Autodesk Inventor part; units mm, degrees
ref_plane "Arbeitsebene3" through (-32.75, 5, -38) normal (0, 1, 0) x (0, 0, 1)
ref_plane "YZ Plane" through (0, 0, 0) normal (1, 0, 0) x (0, 1, 0)
ref_plane "XZ Plane" through (0, 0, 0) normal (0, 1, 0) x (-1, 0, 0)
sketch "Skizze1" plane through (0, 0, 0) normal (0, 1, 0) x (-1, 0, 0)
  line L0 (-37.75, -63.9) -> (37.75, -63.9)
  line L1 (42.75, -58.9) -> (42.75, 58.9)
  line L2 (37.75, 63.9) -> (-37.75, 63.9)
  line L3 (-42.75, 58.9) -> (-42.75, -58.9)
  line L4 (-42.75, -63.9) -> (42.75, 63.9) construction
  line L5 (42.75, -63.9) -> (-42.75, 63.9) construction
  arc A0 (42.75, 58.9) -> (37.75, 63.9) centre (37.75, 58.9) ccw
  arc A1 (-37.75, 63.9) -> (-42.75, 58.9) centre (-37.75, 58.9) ccw
  arc A2 (-42.75, -58.9) -> (-37.75, -63.9) centre (-37.75, -58.9) ccw
  arc A3 (37.75, -63.9) -> (42.75, -58.9) centre (37.75, -58.9) ccw
  point P0 (0, 0)
  dimension "d0" = 85.5
  dimension "d1" = 127.8
  dimension "d2" = 5
extrude "Extrusion1" add sketch "Skizze1" along normal blind 10
ref_plane "Arbeitsebene1" through (37.75, 0, 0) normal (0, 0, -1) x (-1, 0, 0)
ref_plane "Arbeitsebene2" through (0, 0, 58.9) normal (1, 0, 0) x (0, 0, -1)
sketch "Skizze2" plane through (0, 10, 0) normal (0, 1, 0) x (1, 0, 0)
  line L0 (-12.95, 38) -> (-38.75, 38)
  line L1 (-38.75, -38) -> (-12.95, -38)
  line L2 (-12.95, -38) -> (-12.95, -2.5)
  line L3 (-38.75, 38) -> (-38.75, -38)
  line L4 (-38.75, -38) -> (-12.95, -38)
  line L5 (-12.95, -38) -> (-12.95, 38)
  line L6 (-12.95, 38) -> (-38.75, 38)
  line L7 (-38.75, 38) -> (-38.75, -38)
  line L8 (-11.95, 39) -> (-11.95, -39)
  line L9 (-11.95, -39) -> (-39.75, -39)
  line L10 (-39.75, -39) -> (-39.75, 39)
  line L11 (-39.75, 39) -> (-11.95, 39)
  line L12 (-38.75, 38) -> (-38.75, 39)
  line L13 (-38.75, -38) -> (-38.75, -39)
  point P0 (0, 0)
  dimension "d5" = 1
extrude "Extrusion2" cut sketch "Skizze2" against normal through all contours L5 L2 L1 L3 L0 | L0 L12 L11 L8 L9 L13 L1 L2 L5
ref_plane "Arbeitsebene3" through (-32.75, 5, -38) normal (0, 1, 0) x (0, 0, 1)
sketch "Skizze3" plane through (0, 10, 0) normal (0, 1, 0) x (1, 0, 0)
  line L0 (-11.95, -39) -> (-38.75, -39)
  line L1 (-38.75, 39) -> (-11.95, 39)
  line L2 (-11.95, 39) -> (-11.95, -39)
  arc A0 (-37.75, 63.9) -> (-42.75, 58.9) centre (-37.75, 58.9) ccw
  line L3 (-42.75, 58.9) -> (-42.75, -58.9)
  arc A1 (-42.75, -58.9) -> (-37.75, -63.9) centre (-37.75, -58.9) ccw
  line L4 (-37.75, -63.9) -> (37.75, -63.9)
  arc A2 (37.75, -63.9) -> (42.75, -58.9) centre (37.75, -58.9) ccw
  line L5 (42.75, -58.9) -> (42.75, 58.9)
  arc A3 (42.75, 58.9) -> (37.75, 63.9) centre (37.75, 58.9) ccw
  line L6 (37.75, 63.9) -> (-37.75, 63.9)
  line L7 (-39.75, -39) -> (-39.75, 39)
  line L8 (-11.95, 39) -> (-11.95, -39)
  line L9 (-39.75, -39) -> (-11.95, -39)
  line L10 (-11.95, -39) -> (-11.95, -34)
  line L11 (-11.95, -34) -> (-39.75, -34)
  line L12 (-39.75, -34) -> (-39.75, -39)
  line L13 (-39.75, 39) -> (-11.95, 39)
  line L14 (-11.95, 39) -> (-11.95, 34)
  line L15 (-11.95, 34) -> (-39.75, 34)
  line L16 (-39.75, 34) -> (-39.75, 39)
  line L17 (-38.75, -39) -> (-38.75, 39)
  point P0 (0, 0)
  point P1 (-11.95, -34)
  point P2 (-38.75, 34)
  point P3 (-38.75, -34)
  dimension "d8" = 27.8
  dimension "d9" = 5
  dimension "d10" = 5
extrude "Extrusion3" add sketch "Skizze3" against normal blind 1 contours L0 L17 L11 L2 | L15 L17 L1 L2
sketch "Skizze4" plane through (0, 0, 0) normal (0, -1, 0) x (1, 0, 0)
  line L0 (-38.75, 39) -> (-11.95, 39)
  line L1 (-11.95, 39) -> (-11.95, -39)
  line L2 (-11.95, -39) -> (-38.75, -39)
  arc A0 (-42.75, -58.9) -> (-37.75, -63.9) centre (-37.75, -58.9) ccw
  line L3 (37.75, -63.9) -> (-37.75, -63.9)
  arc A1 (37.75, -63.9) -> (42.75, -58.9) centre (37.75, -58.9) ccw
  line L4 (42.75, 58.9) -> (42.75, -58.9)
  arc A2 (42.75, 58.9) -> (37.75, 63.9) centre (37.75, 58.9) ccw
  line L5 (-37.75, 63.9) -> (37.75, 63.9)
  arc A3 (-37.75, 63.9) -> (-42.75, 58.9) centre (-37.75, 58.9) ccw
  line L6 (-42.75, -58.9) -> (-42.75, 58.9)
  line L7 (-11.95, -34) -> (-11.95, 34)
  line L8 (-11.95, 34) -> (12.75, 34)
  line L9 (12.75, 34) -> (12.75, -34)
  line L10 (12.75, -34) -> (-11.95, -34)
  line L11 (-11.95, -34) -> (-11.95, 34)
  line L12 (-2.45, 7.5) -> (-2.45, -8)
  line L13 (12.75, -34.1) -> (12.75, -39.1)
  line L14 (-38.75, -39) -> (-38.75, 39)
  point P0 (0, 0)
  point P1 (-11.95, -34)
  dimension "d14" = 5
  dimension "d15" = 5
  dimension "d44" = 0
extrude "Extrusion4" cut sketch "Skizze4" against normal through all contours L8 L9 L10 L1
sketch "Skizze5" plane through (0, 0, 0) normal (0, -1, 0) x (1, 0, 0)
  arc A0 (-42.75, -58.9) -> (-37.75, -63.9) centre (-37.75, -58.9) ccw
  line L0 (37.75, -63.9) -> (-37.75, -63.9)
  arc A1 (37.75, -63.9) -> (42.75, -58.9) centre (37.75, -58.9) ccw
  line L1 (42.75, 58.9) -> (42.75, -58.9)
  arc A2 (42.75, 58.9) -> (37.75, 63.9) centre (37.75, 58.9) ccw
  line L2 (-37.75, 63.9) -> (37.75, 63.9)
  arc A3 (-37.75, 63.9) -> (-42.75, 58.9) centre (-37.75, 58.9) ccw
  line L3 (-42.75, -58.9) -> (-42.75, 58.9)
  line L4 (-11.95, 34) -> (12.75, 34)
  line L5 (12.75, 34) -> (12.75, -34)
  line L6 (12.75, -34) -> (-11.95, -34)
  line L7 (-11.95, -34) -> (-11.95, -39)
  line L8 (-11.95, -39) -> (-38.75, -39)
  line L9 (-38.75, 39) -> (-11.95, 39)
  line L10 (-11.95, 39) -> (-11.95, 34)
  circle A4 centre (-19.85, -47) radius 1.4
  circle A5 centre (-19.85, 47) radius 1.4
  line L11 (-38.75, -39) -> (-38.75, 39)
  circle A6 centre (-33.9798, 47) radius 1.4
  circle A7 centre (-33.9798, -47) radius 1.4
  circle A8 centre (-8.45, -42) radius 1.4
  point P0 (0, 0)
  dimension "d18" = 2.8
  dimension "d19" = 2.8
  dimension "d20" = 8
  dimension "d21" = 8
  dimension "d45" = 2.8
  dimension "d46" = 2.8
  dimension "d47" = 2.8
  dimension "d48" = 8
  dimension "d49" = 3.5
extrude "Extrusion5" cut sketch "Skizze5" against normal through all contours A4 | A5 | A6 | A7 | A8
sketch "Skizze9" plane through (0, 9, 0) normal (0, -1, 0) x (1, 0, 0)
  circle A0 centre (-19.85, 47) radius 1.4
  circle A1 centre (-19.85, -47) radius 1.4
  arc A2 (-42.75, -58.9) -> (-37.75, -63.9) centre (-37.75, -58.9) ccw
  line L0 (37.75, -63.9) -> (-37.75, -63.9)
  arc A3 (37.75, -63.9) -> (42.75, -58.9) centre (37.75, -58.9) ccw
  line L1 (42.75, 58.9) -> (42.75, -58.9)
  arc A4 (42.75, 58.9) -> (37.75, 63.9) centre (37.75, 58.9) ccw
  line L2 (-37.75, 63.9) -> (37.75, 63.9)
  arc A5 (-37.75, 63.9) -> (-42.75, 58.9) centre (-37.75, 58.9) ccw
  line L3 (-42.75, -58.9) -> (-42.75, 58.9)
  line L4 (12.75, 34) -> (12.75, -34)
  line L5 (12.75, -34) -> (-11.95, -34)
  line L6 (-11.95, -34) -> (-11.95, -39)
  line L7 (-11.95, -39) -> (-38.75, -39)
  line L8 (-38.75, 39) -> (-11.95, 39)
  line L9 (-11.95, 39) -> (-11.95, 34)
  line L10 (-11.95, 34) -> (12.75, 34)
  line L11 (-38.75, 39) -> (-11.95, 39)
  line L12 (-39.75, 39) -> (-11.95, 39)
  line L13 (-11.95, 39) -> (-11.95, 34)
  line L14 (-11.95, 34) -> (-39.75, 34)
  line L15 (-39.75, 34) -> (-39.75, 39)
  line L16 (-11.95, -39) -> (-38.75, -39)
  line L17 (-39.75, -39) -> (-39.75, -34)
  line L18 (-11.95, -39) -> (-39.75, -39)
  line L19 (-39.75, -39) -> (-39.75, -34)
  line L20 (-39.75, -34) -> (-11.95, -34)
  line L21 (-11.95, -34) -> (-11.95, -39)
  line L22 (-38.75, -39) -> (-38.75, 39)
  point P0 (0, 0)
  point P1 (-38.75, 34)
  point P2 (-38.75, -34)
extrude "Extrusion8" add sketch "Skizze9" along normal blind 0.6 contours L14 L22 L8 L9 | L6 L7 L22 L20 | L14 L15 L12 L22
sketch "Skizze10" plane through (0, 10, 0) normal (0, 1, 0) x (1, 0, 0)
  line L0 (23.25, -52.9) -> (23.25, 33.1)
  line L1 (23.25, -52.9) -> (14.45, -52.9)
  line L2 (14.45, -52.9) -> (14.45, 33.1)
  line L3 (14.45, 33.1) -> (23.25, 33.1)
  circle A0 centre (19.25, -37.4) radius 3.25
  circle A1 centre (19.25, 17.6) radius 3.25
  line L4 (41.05, -52.9) -> (41.05, 33.1)
  line L5 (41.05, -52.9) -> (32.25, -52.9)
  line L6 (32.25, -52.9) -> (32.25, 33.1)
  line L7 (32.25, 33.1) -> (41.05, 33.1)
  circle A2 centre (36.25, -37.4) radius 3.25
  circle A3 centre (36.25, 17.6) radius 3.25
  point P0 (0, 0)
hole "Bohrung2" at (36.25, 10, 37.4) at (36.25, 10, -17.6) at (19.25, 10, 37.4) at (19.25, 10, -17.6) direction (0, -1, 0) diameter 2.8 end through all counterbore diameter 6.5 counterbore depth 4
properties part number "TIRFImager_base_v0"
Check sheet for the modelled part. Datum: model origin and axes. Units: mm. A direction names the side the tool comes from. Give positions to 0.01 mm unless a question says otherwise; leave off trailing zeros. Loops run counter-clockwise (first coordinate to the right, second up) from the corner with the lowest first, then second, coordinate; pieces in that order, holes last. Notation, with made-up numbers: M 67.25,65.5 L 92.25,65.5 A6 ccw 92.25,74.5 Z; hole C 43,32 d3. An arc over 180 degrees is marked long. Answer in a Markdown table with one row per item.
1) Mould release check, pull along Z, two halves, no side actions. Record for faces 4 (the face through (42.75, 5, 1)), 5 (the face through (20.617, 2.958, 37.097)), 6 (the face through (-41.32, 4.93, -62.4)): released by +Z, released by -Z, zero draft, split by the parting line, or undercut.
Solutions:
| item | result |
|---|---|
| face 4 | zero draft |
| face 5 | undercut |
| face 6 | released by -Z |
2) Thickness scan on line 1 (Z direction, x = 36.25, y = 1.2); line 2 (X direction, y = 7.95, z = 37.4); line 3 (X direction, y = 2.15, z = -17.6). Record the ranges inside material, lowest first.
Solutions:
| item | result |
|---|---|
| line 1 | z = -63.9 to -19, -16.2 to 36, 38.8 to 63.9 |
| line 2 | x = -42.75 to -38.75, -11.95 to 16, 22.5 to 33, 39.5 to 42.75 |
| line 3 | x = -42.75 to -38.75, 12.75 to 17.85, 20.65 to 34.85, 37.65 to 42.75 |
3) Tool access check on faces 1 (the face through (-26, 8.4, 37)), 2 (the face through (12.75, 5, 0)), 3 (the face through (37, 6, 39)). Record the directions out of +Z, -Z, +X, -X, +Y, -Y that give a thin tool (end or side, any length) a straight path to the whole face; none if there is none.
Solutions:
| item | result |
|---|---|
| face 1 | -Y |
| face 2 | +Y, -Y |
| face 3 | +Y |
4) Cross-section at D-D (y = 2). Count the separate pieces of the cut face and the enclosed holes in it, plus the area to 3 significant figures.
Solutions:
| item | result |
|---|---|
| separate pieces | 1 |
| enclosed holes | 10 |
| area | 7,080 mm^2 |
5) Depth check by flat-ended pin: pin 1 (5 mm diameter, centred on x = 36.25, z = -17.6, fed in from +Y); pin 2 (5.5 mm diameter, centred on x = -28, z = 35.5, fed in from -Y). Enter the tip coordinate at first touch or a pass-through.
Solutions:
| item | result |
|---|---|
| pin 1 | stops at y = 6 |
| pin 2 | stops at y = 8.4 |
6) Cross-section at A-A (x = -4). Enter the section's corners in (y, z), plus the area to 3 significant figures.
Solutions:
| item | result |
|---|---|
| outline | M 0,-63.9 L 10,-63.9 L 10,-34 L 0,-34 Z; M 0,34 L 10,34 L 10,63.9 L 0,63.9 Z |
| area | 598 mm^2 |
7) Cross-section at C-C (z = 37.4). Enter the section's corners in (x, y), plus the area to 3 significant figures.
Solutions:
| item | result |
|---|---|
| outline | M -42.75,0 L -38.75,0 L -38.75,8.4 L -11.95,8.4 L -11.95,0 L 17.85,0 L 17.85,6 L 16,6 L 16,10 L -42.75,10 Z; M 20.65,0 L 34.85,0 L 34.85,6 L 33,6 L 33,10 L 22.5,10 L 22.5,6 L 20.65,6 Z; M 37.65,0 L 42.75,0 L 42.75,10 L 39.5,10 L 39.5,6 L 37.65,6 Z |
| area | 544 mm^2 |
8) Cross-section at B-B (z = -42). Enter the section's corners in (x, y), plus the area to 3 significant figures.
Solutions:
| item | result |
|---|---|
| outline | M -42.75,0 L -9.85,0 L -9.85,10 L -42.75,10 Z; M -7.05,0 L 42.75,0 L 42.75,10 L -7.05,10 Z |
| area | 827 mm^2 |
